Could you check a few things on this model? Use its own coordinates, in mm. Round coordinates to 2 decimals unless told otherwise and drop trailing zeros. Order: outer loops, then holes, each group sorted by start corner. A loop starts at its lowest first (then second) coordinate and runs counter-clockwise, first axis right, second up. Notation, with made-up numbers: (-17, -1.75) - (16, -1.75) arc R11 ccw to (16, 10.25) - close; hole circle Ø6 at (-24.75, -13). An arc over 180 degrees is marked (long way). Return JSON: item names as keys, results as strings. Group by question number.
from build123d import *

# Parameters (mm, degrees)
EXTRUDE_1_DEPTH    = 4
HOLE_WIZARD_M5_1_D = 4.2


with BuildPart() as part:
    # 草图1 → 凸台-拉伸1 (new body)
    with BuildSketch(Plane(origin=(0, 0, 0), x_dir=(1, 0, 0), z_dir=(0, 1, 0))):
        Polygon((4.618802154, 0), (2.309401077, 4), (-2.309401077, 4), (-4.618802154, 0), (-2.309401077, -4), (2.309401077, -4), align=None)
    extrude(amount=EXTRUDE_1_DEPTH)

    # M5 螺纹孔1 (through all)
    with Locations(Plane(origin=(0, 4, 0), x_dir=(1, 0, 0), z_dir=(0, 1, 0))):
        with Locations((0, 0)):
            Hole(HOLE_WIZARD_M5_1_D / 2)

    # 草图4 → 切除-旋转1 (revolve, cut)
    with BuildSketch(Plane(origin=(0, 0, 0), x_dir=(0, 0, -1), z_dir=(1, 0, 0)), mode=Mode.PRIVATE) as cut_revolve_1_sk:
        Polygon((4, 4), (5.578280707, 3.577100959), (4.847725581, 6.644234984), align=None)
        Polygon((4.847725581, -2.644234984), (4, 0), (5.578280707, 0.422899041), align=None)
    revolve(cut_revolve_1_sk.sketch.rotate(Axis((0, 0, 0), (0, -1, 0)), 180), axis=Axis((0, 0, 0), (0, -1, 0)), mode=Mode.SUBTRACT)


solid = part.part
1) If I drill on line 1 along Z through (x, y) = (1.25, 1.5); line 2 along X through (y, z) = (1.05, 1); line 3 along X through (y, z) = (0.75, 0.5), over which ranges is the centre line in solid material (lowest first)? Write a range as from..to.
2) I want a section at A-A, the plane y = 0.85. List the corners of the cut face in (x, z) for me.
3) We'd pull the mould along Z, two halves only. Please class faces 1 (the conical face through (4.15, 0.04, -0.01)), 2 (the flat face through (2, 4, 2)), 3 (the cylindrical face through (-2.003, 1.972, -0.631)), 4 (the conical face through (2.08, 3.96, 3.59)): +Z half, -Z half, draft (parallel to the pull), parting line (faces both ways), or undercut.
Outcome:
{
 "1": {"line 1": "-4..-1.69, 1.69..4", "line 2": "-4.04..-1.85, 1.85..4.04", "line 3": "-4.33..-2.04, 2.04..4.33"},
 "2": {"outline": "(-4.62, 0) - (-2.31, -4) - (2.31, -4) - (4.62, 0) - (2.31, 4) - (-2.31, 4) - close; hole circle Ø4.2 at (0, 0)"},
 "3": {"face 1": "parting line", "face 2": "draft", "face 3": "undercut", "face 4": "+Z half"}
}
